Drawing for the job (mm, zero at the part's lowest x, y, z). A direction names the side the tool comes from. Coordinates: 2 decimals unless noted, no trailing zeros. Write each loop counter-clockwise with the first axis right and the second up, starting at its lowest first coordinate (ties: lowest second). Pieces come first, ordered by that corner, then holes. Notation, with made-up numbers: M -6,1 L 30,1 A33 ccw 30,31 Z; hole C 54,71 d8. An arc over 180 degrees is marked long. Put each result on its own line as item: value. Start each with the question number.
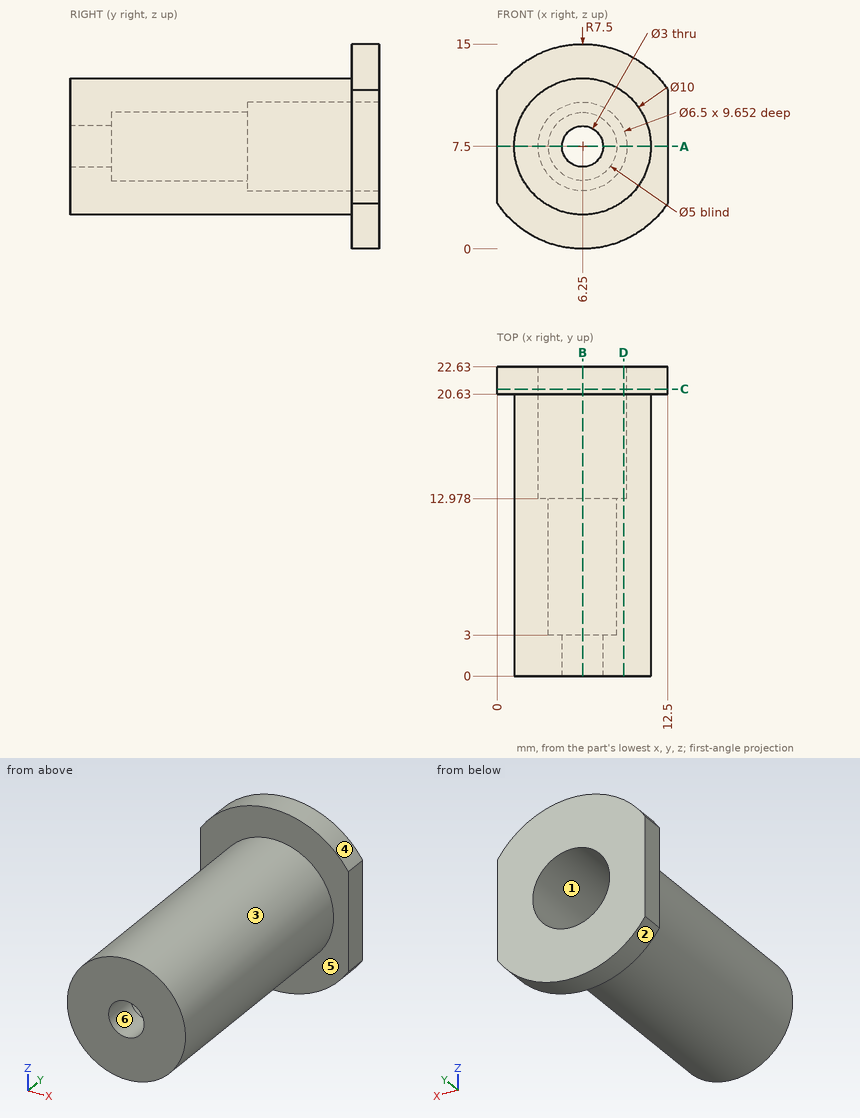
(1) Slice it at B-B, the plane x = 6.25. Write the cut outline in (y, z), then the cut area to 3 significant figures.
(2) Slice it at A-A, the plane z = 7.5. Write the cut outline in (x, y), then the cut area to 3 significant figures.
(3) Drop flat-ended pins along their axis: pin 1 (2 mm diameter, centred on x = 4.5, y = 4.5, fed in from -Z); pin 2 (8 mm diameter, centred on y = 13, z = 12, fed in from -X); pin 3 (5 mm diameter, centred on y = 5.5, z = 13.5, fed in from +X); pin 4 (7 mm diameter, centred on x = 7, z = 7, fed in from +Y). Give the stop position or say it passes through.
(4) Slice it at C-C, the plane y = 21. Write the cut outline in (x, z), then the cut area to 3 significant figures.
(5) Drill centre lines: line 1 (X direction, y = 19, z = 7.5); line 2 (Y direction, x = 7.5, z = 13.75); line 3 (Y direction, x = 4, z = 5.25). Where is each one in solid material? Low to high. Write a range as [from, to].
(6) Two-plate mould, pull along Z, no slides. Class the marked faces 4, 5 and 6: +Z half, -Z half, draft (parallel to the pull), parting line (faces both ways), or undercut.
(7) Which spindle directions (+Z, -Z, +X, -X, +Y, -Y) get a long thin tool onto all of the face, cutting with end or side? Do the marked faces 1, 2 and 3. Say none if no direction does.
(8) Slice it at D-D, the plane x = 9.25. Write the cut outline in (y, z).
Result set:
1. outline: M 0,2.5 L 20.63,2.5 L 20.63,0 L 22.63,0 L 22.63,4.25 L 12.98,4.25 L 12.98,5 L 3,5 L 3,6 L 0,6 Z; M 0,9 L 3,9 L 3,10 L 12.98,10 L 12.98,10.75 L 22.63,10.75 L 22.63,15 L 20.63,15 L 20.63,12.5 L 0,12.5 Z
1. area: 115 mm^2
2. outline: M 0,20.63 L 1.25,20.63 L 1.25,0 L 4.75,0 L 4.75,3 L 3.75,3 L 3.75,12.98 L 3,12.98 L 3,22.63 L 0,22.63 Z; M 7.75,0 L 11.25,0 L 11.25,20.63 L 12.5,20.63 L 12.5,22.63 L 9.5,22.63 L 9.5,12.98 L 8.75,12.98 L 8.75,3 L 7.75,3 Z
2. area: 110 mm^2
3. pin 1: stops at z = 2.56
3. pin 2: stops at x = 1.28
3. pin 3: stops at x = 9.82
3. pin 4: stops at y = 22.63
4. outline: M 0,3.35 A7.5 ccw 12.5,3.35 L 12.5,11.65 A7.5 ccw 0,11.65 Z; hole C 6.25,7.5 d6.5
4. area: 129 mm^2
5. line 1: x = [1.25, 3], [9.5, 11.25]
5. line 2: y = [20.63, 22.63]
5. line 3: y = [0, 12.98]
6. face 4: +Z half
6. face 5: draft
6. face 6: undercut
7. face 1: +Y
7. face 2: -Z, +Y, -Y
7. face 3: -Y
8. outline: M 0,3.5 L 20.63,3.5 L 20.63,0.63 L 22.63,0.63 L 22.63,6.25 L 12.98,6.25 L 12.98,8.75 L 22.63,8.75 L 22.63,14.37 L 20.63,14.37 L 20.63,11.5 L 0,11.5 Z
